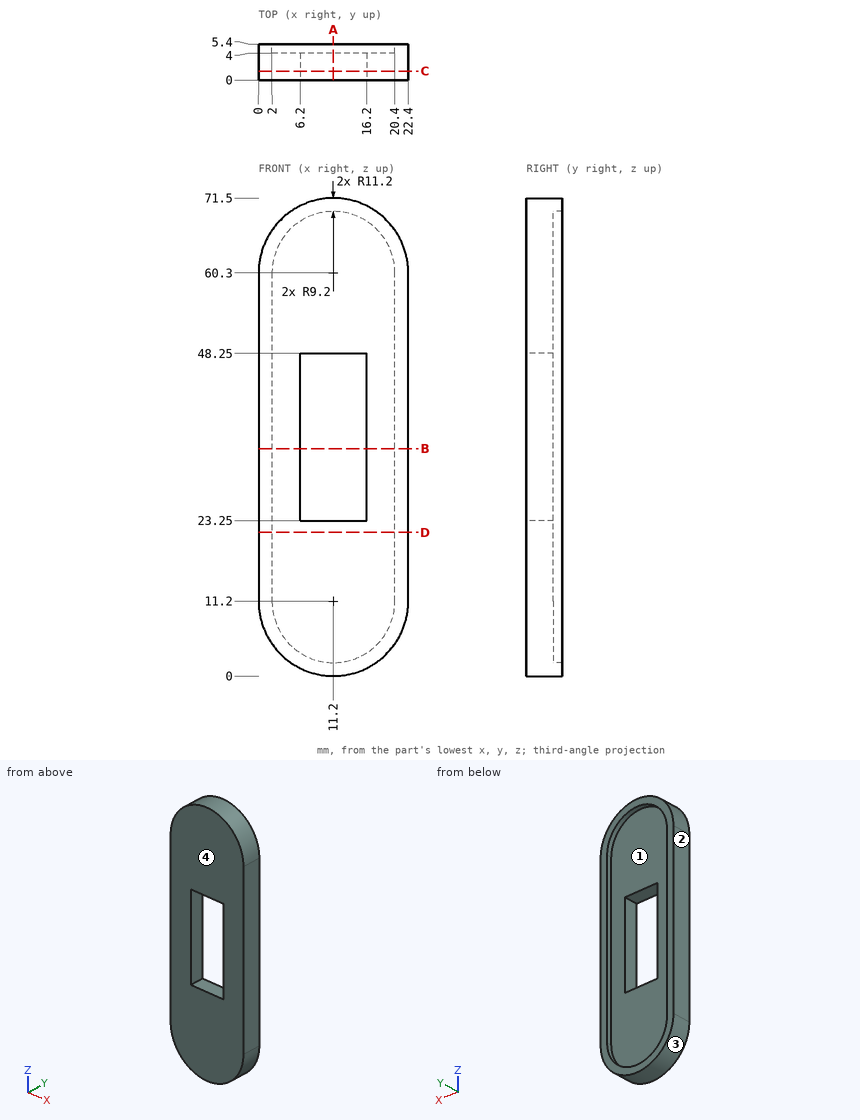
Source: three-view drawing plus pictorial views. Frame: mm from the lowest corner of the part. Coordinates: 2 decimals unless noted, no trailing zeros. Order: outer loops, then holes, each group sorted by start corner. A loop starts at its lowest first (then second) coordinate and runs counter-clockwise, first axis right, second up. Notation, with made-up numbers: (41, 18.25) -> (89, 18.25) arc R24 cw to (89, 44.25) -> close; hole circle Ø3 at (45, -2). An arc over 180 degrees is marked (long way). Write item = value, one per line.
(1) Pin query (flat end, axial travel): pin 1 Ø4 at (x, z) = (20, 30.5) entering from -Y; pin 2 Ø2 at (x, y) = (19, 3) entering from -Z. Return the tip coordinate at first contact, or that it passes through.
Solved:
pin_1 = 0
pin_2 = 2.3
(2) Cut plane A-A on x = 11.2. Return loops of the section in (y, z), plus the area to 3 significant figures.
Solved:
outline = (0, 0) -> (5.4, 0) -> (5.4, 2) -> (4, 2) -> (4, 23.25) -> (0, 23.25) -> close; (0, 48.25) -> (4, 48.25) -> (4, 69.5) -> (5.4, 69.5) -> (5.4, 71.5) -> (0, 71.5) -> close
area = 192 mm²
(3) Pull-direction query (X, two-part tool) for the marked faces 1, 2, 3 and 4; classes: pulls with the +X half, pulls with the -X half, needs draft (parallel to the pull), parting line crosses it, or undercut.
Solved:
face_1 = undercut
face_2 = pulls with the -X half
face_3 = parting line crosses it
face_4 = needs draft
(4) Cut plane B-B on z = 34. Return loops of the section in (x, y), plus the area to 3 significant figures.
Solved:
outline = (0, 0) -> (6.2, 0) -> (6.2, 4) -> (2, 4) -> (2, 5.4) -> (0, 5.4) -> close; (16.2, 0) -> (22.4, 0) -> (22.4, 5.4) -> (20.4, 5.4) -> (20.4, 4) -> (16.2, 4) -> close
area = 55.2 mm²
(5) Cut plane C-C on y = 1.35. Return loops of the section in (x, z), plus the area to 3 significant figures.
Solved:
outline = (0, 11.2) arc R11.2 ccw to (22.4, 11.2) -> (22.4, 60.3) arc R11.2 ccw to (0, 60.3) -> close; hole (6.2, 23.25) -> (16.2, 23.25) -> (16.2, 48.25) -> (6.2, 48.25) -> close
area = 1,240 mm²
(6) Cut plane D-D on z = 21.5. Return loops of the section in (x, y).
Solved:
outline = (0, 0) -> (22.4, 0) -> (22.4, 5.4) -> (20.4, 5.4) -> (20.4, 4) -> (2, 4) -> (2, 5.4) -> (0, 5.4) -> close
(7) Line query: line 1 (Z direction, x = 11.25, y = 2.5); line 2 (X direction, y = 2.1, z = 25); line 3 (X direction, y = 4.45, z = 14). Output: solid intervals per line, ascending.
Solved:
line_1 = 0 to 23.25, 48.25 to 71.5
line_2 = 0 to 6.2, 16.2 to 22.4
line_3 = 0 to 2, 20.4 to 22.4
